Read the model definition and answer for the solid it produces. Units are mm, in the model's axes. Coordinates: 2 decimals unless noted, no trailing zeros. Order: outer loops, then holes, each group sorted by start corner. A loop starts at its lowest first (then second) coordinate and runs counter-clockwise, first axis right, second up. Notation, with made-up numbers: (-14, -30) - (35, -30) arc R22 cw to (35, 9) - close; hole circle Ø6 at (-35.75, -39). An arc over 180 degrees is marked (long way). Write item = value, one per line.
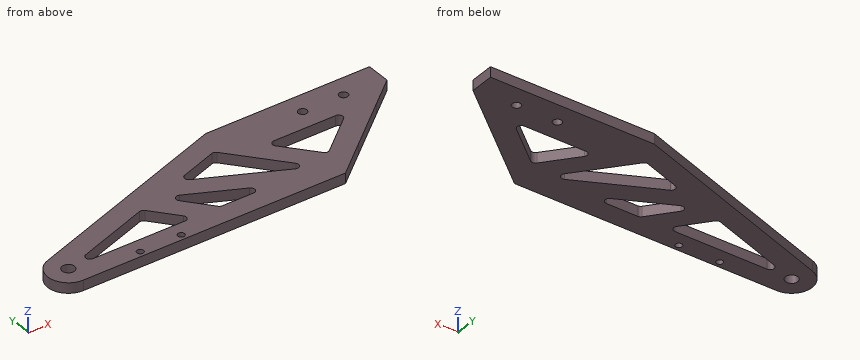
from build123d import *

# Parameters (mm, degrees)
EXTRUDE_1_DEPTH         = 5
SKETCH_2_R              = 3
CUT_EXTRUDE_1_DEPTH     = 198.863589374
CUT_EXTRUDE_2_DEPTH     = 198.863589374
HOLE_WIZARD_3_2_3_2_1_D = 3.2
HOLE_WIZARD_4_2_4_2_1_D = 4.2
CUT_EXTRUDE_3_DEPTH     = 198.863589374


with BuildPart() as part:
    # 草图1 → 凸台-拉伸1 (new body)
    with BuildSketch(Plane.XY):
        with BuildLine():
            Line((0, 0), (0, 55))
            Line((0, 55), (-80, 55))
            Line((-80, 55), (-183.254947339, 19.455438531))
            ThreePointArc((-183.254947339, 19.455438531), (-189.862920088, 8.349906868), (-180, 0))
            Line((-180, 0), (0, 0))
        make_face()
    extrude(amount=EXTRUDE_1_DEPTH)

    # 草图2 → 切除-拉伸1 (cut, through all)
    with BuildSketch(Plane.XY.offset(5)):
        with Locations((-180, 10)):
            Circle(SKETCH_2_R)
    extrude(amount=-CUT_EXTRUDE_1_DEPTH, mode=Mode.SUBTRACT)

    # 草图3 → 切除-拉伸2 (cut, through all)
    with BuildSketch(Plane.XY.offset(5)):
        with BuildLine():
            Line((-113.975045622, 26.000798899), (-88.692623676, 13.801264258))
            ThreePointArc((-88.692623676, 13.801264258), (-87.612105141, 11.554202129), (-89.561788258, 10))
            Line((-89.561788258, 10), (-104.866847196, 10))
            ThreePointArc((-104.866847196, 10), (-105.72348841, 10.192746329), (-106.415015174, 10.733834169))
            Line((-106.415015174, 10.733834169), (-116.392378182, 22.93336881))
            ThreePointArc((-116.392378182, 22.93336881), (-116.415051775, 25.437459016), (-113.975045622, 26.000798899))
        make_face()
        with BuildLine():
            Line((-168.696609563, 13.891087706), (-133.510036225, 26.003740428))
            ThreePointArc((-133.510036225, 26.003740428), (-132.31236206, 26.036486353), (-131.310878779, 25.378818552))
            Line((-131.310878779, 25.378818552), (-121.40457196, 13.266165831))
            ThreePointArc((-121.40457196, 13.266165831), (-121.145486268, 11.143358786), (-122.952739938, 10))
            Line((-122.952739938, 10), (-168.045620095, 10))
            ThreePointArc((-168.045620095, 10), (-170.018204112, 11.669981374), (-168.696609563, 13.891087706))
        make_face()
        with BuildLine():
            Line((-10, 30.729916775), (-10, 12))
            ThreePointArc((-10, 12), (-10.585786438, 10.585786438), (-12, 10))
            Line((-12, 10), (-34.47590013, 10))
            ThreePointArc((-34.47590013, 10), (-36.356443285, 11.319149472), (-35.756268929, 13.536442559))
            Line((-35.756268929, 13.536442559), (-13.280368799, 32.266359334))
            ThreePointArc((-13.280368799, 32.266359334), (-11.151689208, 32.541095617), (-10, 30.729916775))
        make_face()
        with BuildLine():
            Line((-61.350416127, 35), (-31.144599222, 35))
            ThreePointArc((-31.144599222, 35), (-29.264056067, 33.680850528), (-29.864230423, 31.463557441))
            Line((-29.864230423, 31.463557441), (-47.69061417, 16.608237652))
            ThreePointArc((-47.69061417, 16.608237652), (-49.152054461, 16.152893798), (-50.507425528, 16.864311412))
            Line((-50.507425528, 16.864311412), (-62.886858686, 31.719631201))
            ThreePointArc((-62.886858686, 31.719631201), (-63.161594969, 33.848310792), (-61.350416127, 35))
        make_face()
        with BuildLine():
            Line((-84.16091357, 41.62799771), (-63.717267008, 17.095621836))
            ThreePointArc((-63.717267008, 17.095621836), (-63.677184734, 14.584574586), (-66.12287415, 14.013988778))
            Line((-66.12287415, 14.013988778), (-104.307462185, 32.43920949))
            ThreePointArc((-104.307462185, 32.43920949), (-105.434815281, 34.358444754), (-104.08928707, 36.131561455))
            Line((-104.08928707, 36.131561455), (-86.348345597, 42.238716617))
            ThreePointArc((-86.348345597, 42.238716617), (-85.15953535, 42.273959311), (-84.16091357, 41.62799771))
        make_face()
    extrude(amount=-CUT_EXTRUDE_2_DEPTH, mode=Mode.SUBTRACT)

    # Ø3.2 (3.2) 直径孔1 (through all)
    with Locations(Plane(origin=(-150, 3, 5), x_dir=(1, 0, 0), z_dir=(0, 0, 1))):
        with Locations((0, 0), (20, 0)):
            Hole(HOLE_WIZARD_3_2_3_2_1_D / 2)

    # Ø4.2 (4.2) 直径孔1 (through all)
    with Locations(Plane(origin=(-40, 45, 5), x_dir=(1, 0, 0), z_dir=(0, 0, 1))):
        with Locations((0, 0), (20, 0)):
            Hole(HOLE_WIZARD_4_2_4_2_1_D / 2)

    # 草图8 → 切除-拉伸3 (cut, through all)
    with BuildSketch(Plane.XY.offset(5)):
        Polygon((0, 0), (0, 43.333333333), (-52, 0), align=None)
    extrude(amount=-CUT_EXTRUDE_3_DEPTH, mode=Mode.SUBTRACT)


solid = part.part
1) Flat-ended cylindrical pins translate along their axes: pin 1 Ø1.5 at (x, z) = (-48.5, 2) entering from -Y; pin 2 Ø2.5 at (x, z) = (-97, 2.5) entering from +Y; pin 3 Ø2.5 at (x, z) = (-141.5, 2.5) entering from +Y. Find the tip coordinate at first contact, or state that the pin passes through.
Returned:
pin_1 = 2.29
pin_2 = 49.58
pin_3 = 34.26
2) The part is cut by section B-B (x = -150). Determine the outline of the cut face in (y, z).
Returned:
outline = (0, 0) - (1.4, 0) - (1.4, 5) - (0, 5) - close; (4.6, 0) - (10, 0) - (10, 5) - (4.6, 5) - close; (20.33, 0) - (30.9, 0) - (30.9, 5) - (20.33, 5) - close
3) The part is cut by section A-A (x = -20). Determine the outline of the cut face in (y, z), and give its area (3 significant figures).
Returned:
outline = (26.67, 0) - (42.9, 0) - (42.9, 5) - (26.67, 5) - close; (47.1, 0) - (55, 0) - (55, 5) - (47.1, 5) - close
area = 121 mm^2
4) Straight lines are drawn through the part: line 1 along Y through (x, z) = (-150, 2); line 2 along Y through (x, z) = (-94.5, 3.35); line 3 along X through (y, z) = (11, 4.2). For each, find the intervals that lie inside material, in ascending order. Write a range as from..to.
Returned:
line_1 = 0..1.4, 4.6..10, 20.33..30.9
line_2 = 0..10, 16.6..27.71, 39.43..50.01
line_3 = -189.95..-182.83, -177.17..-169.78, -121.22..-106.63, -87.83..-38.8
5) The part is cut by section C-C (y = 45). Determine the outline of the cut face in (x, z).
Returned:
outline = (-109.05, 0) - (-42.1, 0) - (-42.1, 5) - (-109.05, 5) - close; (-37.9, 0) - (-22.1, 0) - (-22.1, 5) - (-37.9, 5) - close; (-17.9, 0) - (0, 0) - (0, 5) - (-17.9, 5) - close
6) The part is cut by section D-D (z = 2.95). Count the separate pieces of the cut face and the enclosed holes in it, and give its area (3 significant figures).
Returned:
separate_pieces = 1
enclosed_holes = 9
area = 5,570 mm^2
